Read the model definition and answer for the solid it produces. Units are mm, in the model's axes. Face numbers are marked on the shaded views. A direction names the side the tool comes from. Coordinates: 2 decimals unless noted, no trailing zeros. Write each loop counter-clockwise with the first axis right and the second up, starting at its lowest first coordinate (ties: lowest second). Pieces come first, ordered by that corner, then holes. Notation, with made-up numbers: (74, 1.5) - (129, 1.5) arc R19 cw to (129, 30.5) - close; hole circle Ø8 at (19, 80). An arc over 180 degrees is marked (long way). Use a Markdown table: item, result.
from build123d import *

# Parameters (mm, degrees)
MODEL_R                 = 1.5
SALIENTE_EXTRUIR1_DEPTH = 3


with BuildPart() as part:
    # Model → Saliente-Extruir1 (new body)
    with BuildSketch(Plane.XY):
        with BuildLine():
            Line((180.84213351, 175.823953209), (162.84213351, 175.823953209))
            Line((162.84213351, 175.823953209), (162.84213351, 193.823953209))
            Line((162.84213351, 193.823953209), (167.34213351, 193.823953209))
            ThreePointArc((167.34213351, 193.823953209), (169.064208955, 193.481411105), (170.524114025, 192.505933724))
            Line((170.524114025, 192.505933724), (179.524114025, 183.505933724))
            ThreePointArc((179.524114025, 183.505933724), (180.499591406, 182.046028655), (180.84213351, 180.323953209))
            Line((180.84213351, 180.323953209), (180.84213351, 175.823953209))
        make_face()
        with Locations((176.34213351, 180.323953209)):
            Circle(MODEL_R, mode=Mode.SUBTRACT)
        with BuildLine():
            Line((164.84213351, 181.948953209), (169.84213351, 181.948953209))
            ThreePointArc((169.84213351, 181.948953209), (170.372463595, 181.729283295), (170.59213351, 181.198953209))
            Line((170.59213351, 181.198953209), (170.59213351, 179.448953209))
            ThreePointArc((170.59213351, 179.448953209), (170.372463595, 178.918623123), (169.84213351, 178.698953209))
            Line((169.84213351, 178.698953209), (164.84213351, 178.698953209))
            ThreePointArc((164.84213351, 178.698953209), (164.311803424, 178.918623123), (164.09213351, 179.448953209))
            Line((164.09213351, 179.448953209), (164.09213351, 181.198953209))
            ThreePointArc((164.09213351, 181.198953209), (164.311803424, 181.729283295), (164.84213351, 181.948953209))
        make_face(mode=Mode.SUBTRACT)
        with BuildLine():
            Line((169.041348982, 189.928670304), (172.576882888, 186.393136398))
            ThreePointArc((172.576882888, 186.393136398), (172.796552802, 185.862806312), (172.576882888, 185.332476227))
            Line((172.576882888, 185.332476227), (171.339446021, 184.095039359))
            ThreePointArc((171.339446021, 184.095039359), (170.809115935, 183.875369445), (170.278785849, 184.095039359))
            Line((170.278785849, 184.095039359), (166.743251943, 187.630573265))
            ThreePointArc((166.743251943, 187.630573265), (166.523582029, 188.160903351), (166.743251943, 188.691233437))
            Line((166.743251943, 188.691233437), (167.98068881, 189.928670304))
            ThreePointArc((167.98068881, 189.928670304), (168.511018896, 190.148340218), (169.041348982, 189.928670304))
        make_face(mode=Mode.SUBTRACT)
    extrude(amount=SALIENTE_EXTRUIR1_DEPTH)


solid = part.part
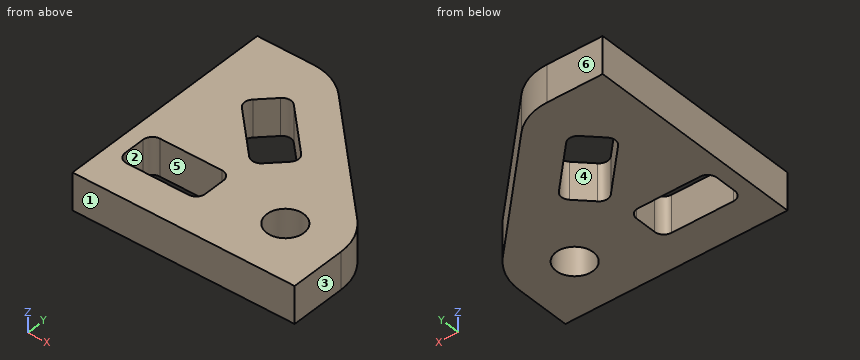
(1) A cutting plane is placed at B-B, the plane y = 179.75. Write down the section's boundary in (x, z).
Report:
| item | result |
|---|---|
| outline | (162.84, 0) - (164.09, 0) - (164.09, 3) - (162.84, 3) - close; (170.59, 0) - (174.96, 0) - (174.96, 3) - (170.59, 3) - close; (177.73, 0) - (180.84, 0) - (180.84, 3) - (177.73, 3) - close |
(2) For the marked faces 1 and 2, determine the directions among +Z, -Z, +X, -X, +Y, -Y from which every point of the face is accessible in a straight line to the end or side of a thin tool.
Report:
| item | result |
|---|---|
| face 1 | +Z, -Z, +X, -X, -Y |
| face 2 | +Z, -Z |
(3) The mould has two halves that part along X. Classify the marked faces 3, 4, 5 and 6: pulls with the +X half, pulls with the -X half, needs draft (parallel to the pull), parting line crosses it, or undercut.
Report:
| item | result |
|---|---|
| face 3 | pulls with the +X half |
| face 4 | undercut |
| face 5 | undercut |
| face 6 | needs draft |
(4) Straight lines are drawn through the part: L1, parallel to Y at x = 166.25, z = 1.4; L2, parallel to Y at x = 170.5, z = 1.9; L3, parallel to Y at x = 169.5, z = 1.6. For each, find the intervals that lie inside material, in ascending order.
Report:
| item | result |
|---|---|
| L1 | y = 175.82 to 178.7, 181.95 to 193.82 |
| L2 | y = 175.82 to 179.09, 181.56 to 183.94, 188.47 to 192.53 |
| L3 | y = 175.82 to 178.7, 181.95 to 184.87, 189.47 to 193.27 |
(5) A cutting plane is placed at D-D, the plane y = 189. Write down the section's boundary in (x, z), and give its area (3 significant figures).
Report:
| item | result |
|---|---|
| outline | (162.84, 0) - (167.05, 0) - (167.05, 3) - (162.84, 3) - close; (169.97, 0) - (174.03, 0) - (174.03, 3) - (169.97, 3) - close |
| area | 24.8 mm² |
(6) This flat-tipped pin is pushed along its axis until it touches: P1, Ø0.9, axis at x = 168, z = 2, coming from the +Y side. Where does it stop, or does it pass through?
Report:
| item | result |
|---|---|
| P1 | stops at y = 193.82 |
(7) A cutting plane is placed at C-C, the plane z = 1.65. Write down the section's boundary in (x, y), and give its area (3 significant figures).
Report:
| item | result |
|---|---|
| outline | (162.84, 175.82) - (180.84, 175.82) - (180.84, 180.32) arc R4.5 ccw to (179.52, 183.51) - (170.52, 192.51) arc R4.5 ccw to (167.34, 193.82) - (162.84, 193.82) - close; hole (164.09, 179.45) arc R0.75 ccw to (164.84, 178.7) - (169.84, 178.7) arc R0.75 ccw to (170.59, 179.45) - (170.59, 181.2) arc R0.75 ccw to (169.84, 181.95) - (164.84, 181.95) arc R0.75 ccw to (164.09, 181.2) - close; hole (166.74, 187.63) - (170.28, 184.1) arc R0.75 ccw to (171.34, 184.1) - (172.58, 185.33) arc R0.75 ccw to (172.58, 186.39) - (169.04, 189.93) arc R0.75 ccw to (167.98, 189.93) - (166.74, 188.69) arc R0.75 ccw to start; hole circle Ø3 at (176.34, 180.32) |
| area | 207 mm² |
(8) A cutting plane is placed at A-A, the plane x = 176. Write down the section's boundary in (y, z).
Report:
| item | result |
|---|---|
| outline | (175.82, 0) - (178.86, 0) - (178.86, 3) - (175.82, 3) - close; (181.78, 0) - (187.03, 0) - (187.03, 3) - (181.78, 3) - close |
